from build123d import *

# Parameters (mm, degrees)
EXTRUDE_1_DEPTH             = 15
HOLE_WIZARD_3_5_3_5_1_D     = 3.5
HOLE_WIZARD_3_5_3_5_1_DEPTH = 4
FILLET_1_R                  = 1
FILLET_2_R                  = 1


with BuildPart() as part:
    # 草图5 → 拉伸-薄壁1 (new body)
    with BuildSketch(Plane(origin=(0, 0, 0), x_dir=(0, 0, -1), z_dir=(1, 0, 0))):
        Polygon((0, -28), (0, 0), (8, 0), (8, -1.2), (1.2, -1.2), (1.2, -28), align=None)
    extrude(amount=EXTRUDE_1_DEPTH)

    # Ø3.5 (3.5) 直径孔1
    with Locations(Plane(origin=(4.305374672, 0, -7.219790434), x_dir=(1, 0, 0), z_dir=(0, 1, 0))):
        with Locations((7.694625328, -2.219790434), (-1.305374672, -2.219790434)):
            Hole(HOLE_WIZARD_3_5_3_5_1_D / 2, depth=HOLE_WIZARD_3_5_3_5_1_DEPTH)

    # 圆角1
    fillet_1_edges = [part.edges().sort_by_distance(p)[0] for p in [
        (15, -28, -0.6),
        (0, -28, -0.6),
        (0, -0.6, -8),
        (15, -0.6, -8),
    ]]
    fillet(fillet_1_edges, radius=FILLET_1_R)

    # 圆角2
    fillet_2_edges = [part.edges().sort_by_distance(p)[0] for p in [
        (7.5, -1.2, -1.2),
        (7.5, 0, 0),
    ]]
    fillet(fillet_2_edges, radius=FILLET_2_R)


solid = part.part
Here's how the part is built. I have some questions about the finished solid (model axes, mm). A direction names the side the tool comes from. Round coordinates to 2 decimals unless told otherwise and drop trailing zeros. Write each loop counter-clockwise with the first axis right and the second up, starting at its lowest first coordinate (ties: lowest second). Pieces come first, ordered by that corner, then holes.
1. I need wall thicknesses on L1, parallel to X at y = -0.7, z = -5; L2, parallel to Z at x = 1, y = -16.25; L3, parallel to Z at x = 12, y = -0.7. Which ranges of each line are inside material? Lowest first, please.
2. Suppose I cut it at B-B (z = -5). List the corners of the cut face in (x, y) for me.
3. For faces 1 (the flat face through (7, -15, -1.2)), 2 (the cylindrical face through (14.715, -0.608, -7.699)), which set-ups out of +Z, -Z, +X, -X, +Y, -Y let a thin tool reach every point of the face, with its end or its side?
4. Will these pins go through, and if not, where does the flat tip stop? pin 1 Ø1 at (x, z) = (2, -6.5) entering from -Y; pin 2 Ø3 at (y, z) = (-4, -4) entering from +X.
5. Suppose I cut it at A-A (x = 3). List the corners of the cut face in (y, z) for me, and give its area (3 significant figures).
6. Suppose I cut it at D-D (y = -5). List the corners of the cut face in (x, z) for me, and give its area (3 significant figures).
7. Suppose I cut it at C-C (x = 6.5). List the corners of the cut face in (y, z) for me, and give its area (3 significant figures).
Answer sheet:
1. L1: x = 0 to 1.25, 4.75 to 10.25, 13.75 to 15
1. L2: z = -1.2 to 0
1. L3: z = -8 to -6.75, -3.25 to -0.05
2. outline: (0, -1.2) - (1.25, -1.2) - (1.25, 0) - (0, 0) - close; (4.75, -1.2) - (10.25, -1.2) - (10.25, 0) - (4.75, 0) - close; (13.75, -1.2) - (15, -1.2) - (15, 0) - (13.75, 0) - close
3. face 1: -Z, +X, -X, -Y
3. face 2: -Z, +X, +Y, -Y
4. pin 1: stops at y = -1.2
4. pin 2: passes through
5. outline: (-28, -1.2) - (-2.2, -1.2) arc R1 cw to (-1.2, -2.2) - (-1.2, -3.25) - (0, -3.25) - (0, -1) arc R1 ccw to (-1, 0) - (-28, 0) - close; (-1.2, -8) - (0, -8) - (0, -6.75) - (-1.2, -6.75) - close
5. area: 37.6 mm2
6. outline: (0, -1.2) - (15, -1.2) - (15, 0) - (0, 0) - close
6. area: 18.0 mm2
7. outline: (-28, -1.2) - (-2.2, -1.2) arc R1 cw to (-1.2, -2.2) - (-1.2, -8) - (0, -8) - (0, -1) arc R1 ccw to (-1, 0) - (-28, 0) - close
7. area: 41.8 mm2
